```python
from build123d import *

# Parameters (mm, degrees)
SKETCH1_R                       = 4.7625
BOSS_EXTRUDE1_DEPTH             = 1.143
BOSS_EXTRUDE2_START             = -1.143
SKETCH2_R                       = 4.0259
BOSS_EXTRUDE2_DEPTH             = 31.75
F_8_32_TAPPED_HOLE1_D           = 3.4544
F_8_32_TAPPED_HOLE1_DEPTH       = 19.05
F_8_32_TAPPED_HOLE1_CSINK_D     = 5.4356
F_8_32_TAPPED_HOLE1_CSINK_ANGLE = 45
F_8_32_TAPPED_HOLE1_TIP         = 1.037806461


with BuildPart() as part:
    # Sketch1 → Boss-Extrude1 (new body)
    with BuildSketch(Plane(origin=(0, 0, 0), x_dir=(1, 0, 0), z_dir=(0, 1, 0))):
        Circle(SKETCH1_R)
    extrude(amount=BOSS_EXTRUDE1_DEPTH)

    # Sketch2 → Boss-Extrude2 (add)
    with BuildSketch(Plane.XZ.offset(BOSS_EXTRUDE2_START)):
        Circle(SKETCH2_R)
    extrude(amount=BOSS_EXTRUDE2_DEPTH)

    # #8-32 Tapped Hole1
    with Locations(Plane(origin=(0, -30.607, 0), x_dir=(-1, 0, 0), z_dir=(0, -1, 0))):
        with Locations((0, 0)):
            CounterSinkHole(F_8_32_TAPPED_HOLE1_D / 2, F_8_32_TAPPED_HOLE1_CSINK_D / 2, depth=F_8_32_TAPPED_HOLE1_DEPTH, counter_sink_angle=F_8_32_TAPPED_HOLE1_CSINK_ANGLE)
            with Locations((0, 0, -(F_8_32_TAPPED_HOLE1_DEPTH + F_8_32_TAPPED_HOLE1_TIP / 2))):  # 118° drill point
                Cone(0, F_8_32_TAPPED_HOLE1_D / 2, F_8_32_TAPPED_HOLE1_TIP, mode=Mode.SUBTRACT)


solid = part.part
```
Work out the finished part from the listing and answer in its coordinate system (mm). A direction names the side the tool comes from. Round coordinates to 2 decimals unless told otherwise and drop trailing zeros. Order: outer loops, then holes, each group sorted by start corner. A loop starts at its lowest first (then second) coordinate and runs counter-clockwise, first axis right, second up.
Q1. Find the intervals of material crossed by line 1 along Z through (x, y) = (0, -21.5); line 2 along Y through (x, z) = (3.5, 3); line 3 along Z through (x, y) = (3.5, -11.5), in increasing order.
Solution:
line 1: z = -4.03 to -1.73, 1.73 to 4.03
line 2: y = 0 to 1.14
line 3: z = -1.99 to 1.99
Q2. Given pin 1 Ø5 at (x, y) = (-1, -10) entering from +Z; pin 2 Ø1 at (x, y) = (2, -24) entering from -Z; pin 3 Ø5 at (y, z) = (-8.5, 0.5) entering from -X, each flat-ended and moving along its own axis, determine where each tip first touches the part or whether it passes through.
Solution:
pin 1: stops at z = 4.03
pin 2: stops at z = -3.74
pin 3: stops at x = -4.03
Q3. The mould has two halves that part along Z. Classify faces 1 (the conical face through (-0.41, -28.6, 1.84)), 2 (the cylindrical face through (-3.78, 0.56, 2.9)), 3 (the flat face through (-2, 0, -4)): pulls with the +Z half, pulls with the -Z half, needs draft (parallel to the pull), parting line crosses it, or undercut.
Solution:
face 1: undercut
face 2: parting line crosses it
face 3: needs draft
Q4. A tool of negligible diameter and unlimited length cuts with its end or side. For faces 4 (the flat face through (1, -30.607, -3)), 5 (the cylindrical face through (-3.195, -15.089, -2.45)), from which of +Z, -Z, +X, -X, +Y, -Y can it reach the whole face along a straight path? Write none if from no direction.
Solution:
face 4: +Z, -Z, +X, -X, -Y
face 5: -Y
Q5. A cutting plane is placed at A-A, the plane x = -3.25. Determine the outline of the cut face in (y, z).
Solution:
outline: (-30.61, -2.38) - (0, -2.38) - (0, -3.48) - (1.14, -3.48) - (1.14, 3.48) - (0, 3.48) - (0, 2.38) - (-30.61, 2.38) - close
Q6. A cutting plane is placed at B-B, the plane z = -3. Determine the outline of the cut face in (x, y).
Solution:
outline: (-3.7, 0) - (-2.68, 0) - (-2.68, -30.61) - (2.68, -30.61) - (2.68, 0) - (3.7, 0) - (3.7, 1.14) - (-3.7, 1.14) - close
Q7. A cutting plane is placed at C-C, the plane y = -22. Determine the outline of the cut face in (x, z).
Solution:
outline: circle Ø8.05 at (0, 0); hole circle Ø3.45 at (0, 0)
